Build history of the part. All positions in model axes, mm. Coordinates: 2 decimals unless noted, no trailing zeros. Write each loop counter-clockwise with the first axis right and the second up, starting at its lowest first coordinate (ties: lowest second). Pieces come first, ordered by that corner, then holes.
Autodesk Inventor part; units mm, degrees
ref_plane "YZ Plane" through (0, 0, 0) normal (1, 0, 0) x (0, 1, 0)
ref_plane "XZ Plane" through (0, 0, 0) normal (0, 1, 0) x (-1, 0, 0)
ref_plane "XY Plane" through (0, 0, 0) normal (0, 0, 1) x (1, 0, 0)
sketch "Sketch1" plane through (0, 0, 0) normal (0, 0, 1) x (1, 0, 0)
  circle A0 centre (-2.6438, 6.9447) radius 6.8758
  line L0 (-9.4616, 7.8359) -> (-6.8245, 12.4034)
  line L1 (-6.8245, 1.4859) -> (-9.4616, 6.0534)
  line L2 (-0.0068, 0.5947) -> (-5.2808, 0.5947)
  line L3 (4.174, 6.0534) -> (1.537, 1.4859)
  line L4 (1.537, 12.4034) -> (4.174, 7.8359)
  line L5 (-5.2808, 13.2947) -> (-0.0068, 13.2947)
  point P0 (0, 0)
  point P1 (1.537, 1.4859)
  dimension "d0" = 13.7516
  dimension "d4" = 360
extrude "Extrusion1" add sketch "Sketch1" along normal blind 111.125 contours A0 L3 L2 L1 L0 L5 L4
sketch "Sketch2" plane through (0, 0, 111.125) normal (0, 0, 1) x (1, 0, 0)
  circle A0 centre (-2.6438, 6.9447) radius 2.5527
  line L0 (-5.2808, 0.5947) -> (-0.0068, 0.5947)
  line L1 (-2.6438, 6.9447) -> (-5.2808, 0.5947) construction
  line L2 (-2.6438, 6.9447) -> (-0.0068, 0.5947) construction
  point P0 (0, 0)
  dimension "d8" = 5.1054
  dimension "d9" = 6.35
extrude "Extrusion2" cut sketch "Sketch2" against normal blind 111.125
equation "\"d6\" = d5"
equation "\"d10\" = d5"
equation "\"d5\" = 111.125"
properties part number "5.5 thundershaft" material "Aluminum 6061"
1. Flat gauge pins, fed straight in: pin 1 (1.5 mm diameter, centred on y = 9.5, z = 81, fed in from -X); pin 2 (4.5 mm diameter, centred on x = -2.64, y = 6.94, fed in from +Z); pin 3 (3 mm diameter, centred on y = 11.5, z = 43, fed in from -X). Where does each tip first touch, or does it go through?
Computed values:
pin 1: stops at x = -8.93
pin 2: passes through
pin 3: stops at x = -8.21
2. Mould opens along Y. For faces 1 (the face through (-3, 13.295, 55)), 2 (the face through (-9.52, 6.93, 54.78)), 3 (the face through (-1.271, 9.097, 56.34)) say: +Y half, -Y half, draft (parallel to the pull), parting line (faces both ways), or undercut.
Computed values:
face 1: +Y half
face 2: parting line
face 3: undercut
3. Saw through at B-B on z = 84.5. List the corners of the cut face in (x, y), plus the area to 3 significant figures.
Computed values:
outline: (-9.46, 6.05) - (-6.82, 1.49) arc R6.88 ccw to (-5.28, 0.59) - (-0.01, 0.59) arc R6.88 ccw to (1.54, 1.49) - (4.17, 6.05) arc R6.88 ccw to (4.17, 7.84) - (1.54, 12.4) arc R6.88 ccw to (-0.01, 13.29) - (-5.28, 13.29) arc R6.88 ccw to (-6.82, 12.4) - (-9.46, 7.84) arc R6.88 ccw to start; hole circle Ø5.11 at (-2.64, 6.94)
area: 117 mm2
4. Saw through at A-A on x = -2.25. List the corners of the cut face in (y, z) (3 decimals).
Computed values:
outline: (0.595, 0) - (4.423, 0) - (4.423, 111.125) - (0.595, 111.125) - close; (9.467, 0) - (13.295, 0) - (13.295, 111.125) - (9.467, 111.125) - close
5. Saw through at D-D on x = 2.5. List the corners of the cut face in (y, z) (3 decimals).
Computed values:
outline: (3.154, 0) - (10.735, 0) - (10.735, 111.125) - (3.154, 111.125) - close
6. Saw through at C-C on y = 10.5. List the corners of the cut face in (x, z) (3 decimals), plus the area to 3 significant figures.
Computed values:
outline: (-7.923, 0) - (2.636, 0) - (2.636, 111.125) - (-7.923, 111.125) - close
area: 1,170 mm2
7. Probe line 1 along X through (y, z) = (7.25, 101.5); line 2 along Y through (x, z) = (0, 81); line 3 along X through (y, z) = (8.75, 63.5). List the from-to ranges inside material, lowest first.
Computed values:
line 1: x = -9.51 to -5.18, -0.11 to 4.23
line 2: y = 0.6 to 13.29
line 3: x = -8.93 to -4.45, -0.84 to 3.65
